Source: CAD feature listing. Evaluate the final solid. Frame: model axes, mm. Face numbers are marked on the shaded views. A direction names the side the tool comes from. Coordinates: 2 decimals unless noted, no trailing zeros. Order: outer loops, then holes, each group sorted by start corner. A loop starts at its lowest first (then second) coordinate and runs counter-clockwise, first axis right, second up. Notation, with made-up numbers: (-7, 44) - (-1, 44) arc R12 cw to (-1, 58) - close; hole circle Ø6 at (47.5, -25.5). An arc over 180 degrees is marked (long way). One line per question, with ' | ' between items.
Autodesk Inventor part; units mm, degrees
ref_plane "YZ Plane" through (0, 0, 0) normal (1, 0, 0) x (0, 1, 0)
ref_plane "XZ Plane" through (0, 0, 0) normal (0, 1, 0) x (-1, 0, 0)
ref_plane "XY Plane" through (0, 0, 0) normal (0, 0, 1) x (1, 0, 0)
sketch "Sketch1" plane through (0, 0, 0) normal (1, 0, 0) x (0, 1, 0)
  circle A0 centre (0, 0) radius 3.175
  circle A1 centre (0, 0) radius 6.35
  dimension "d0" = 6.35
  dimension "d1" = 12.7
extrude "Extrusion1" add sketch "Sketch1" along normal blind 25.4
sketch "Sketch2" plane through (25.4, 0, 0) normal (1, 0, 0) x (0, 0, -1)
  circle A0 centre (0, 0) radius 6.35
  circle A1 centre (0, 0) radius 1.5875
  circle A2 centre (0, 0) radius 6.35
  dimension "d4" = 3.175
extrude "Extrusion2" add sketch "Sketch2" along normal blind 12.7
sketch "Sketch3" plane through (38.1, 0, 0) normal (1, 0, 0) x (0, 0, -1)
  circle A0 centre (0, 0) radius 6.35
  line L0 (2, 16.0268) -> (2, 6.0268)
  line L1 (2, 16.0268) -> (6, 16.0268)
  line L2 (6, 16.0268) -> (6, 2.0791)
  line L3 (-2, 16.0268) -> (-2, 6.0268)
  line L4 (-2, 16.0268) -> (-6, 16.0268)
  line L5 (-6, 16.0268) -> (-6, 2.0791)
  dimension "d11" = 4
  dimension "d12" = 10
  dimension "d13" = 10
extrude "Extrusion3" add sketch "Sketch3" against normal blind 18 contours A0 L0 L1 L2 | L5 L4 L3 A0
chamfer "Chamfer1" distance 9 angle 45 2 edges at (20.1, 16.0268, 4) (20.1, 16.0268, -4)
chamfer "Chamfer2" distance 2 angle 45 2 edges at (38.1, 16.0268, 4) (38.1, 16.0268, -4)
sketch "Sketch5" plane through (20.1, 2.0791, 6) normal (0, 0, 1) x (1, 0, 0)
  line L0 (16, 13.9478) -> (9, 13.9478)
  line L1 (18, 11.9478) -> (18, 0)
  circle A0 centre (13, 8.9478) radius 0.75
  point P0 (-20.1, -2.0791)
  dimension "d30" = 1.5
  dimension "d31" = 5
  dimension "d32" = 5
extrude "Extrusion5" cut sketch "Sketch5" against normal blind 15
sketch "Sketch6" plane through (38.1, 0, 0) normal (1, 0, 0) x (0, 0, -1)
  arc A0 (2, 6.0268) -> (-2, 6.0268) centre (0, 0) ccw
  line L0 (-6, 14.0268) -> (-6, 2.0791)
  line L1 (2, 6.0268) -> (-2, 6.0268)
  point P0 (-6, 3.4641)
extrude "Extrusion6" cut sketch "Sketch6" against normal blind 6
pattern_circular "Circular Pattern3" count 3 over 360 about axis through (0, 0, 0) along (1, 0, 0) of "Extrusion3", "Chamfer2", "Extrusion5", "Extrusion6", "Chamfer1"
sketch "Sketch7" plane through (38.1, 0, 0) normal (1, 0, 0) x (0, 0, -1)
  circle A0 centre (0, 0) radius 1.5875
  circle A1 centre (0, 0) radius 1.524
  line L0 (-1.524, 1.524) -> (1.524, 1.524)
  line L1 (1.524, 1.524) -> (1.524, -1.524)
  line L2 (1.524, -1.524) -> (-1.524, -1.524)
  line L3 (-1.524, -1.524) -> (-1.524, 1.524)
  circle A2 centre (0, 0) radius 1.5875
  dimension "d43" = 3.048
extrude "Extrusion7" add sketch "Sketch7" against normal blind 3.175 contours A0 L1 | L1 A1 L0 A0 | A0 L2 A1 L1 | L0 A0 | A1 | A0 L2 | L0 A1 L3 A0 | L2 A0 L3 A1 | L3 A0
sketch "Sketch8" plane through (38.1, 0, 0) normal (1, 0, 0) x (0, 0, -1)
  line L0 (-1.651, 1.651) -> (1.651, 1.651)
  line L1 (1.651, 1.651) -> (1.651, -1.651)
  line L2 (1.651, -1.651) -> (-1.651, -1.651)
  line L3 (-1.651, -1.651) -> (-1.651, 1.651)
  point P0 (0, 0)
  dimension "d46" = 1.651
  dimension "d48" = 1.651
  dimension "d49" = 3.302
  dimension "d50" = 3.302
extrude "Extrusion8" cut sketch "Sketch8" against normal blind 12.7
properties part number "Coupler"
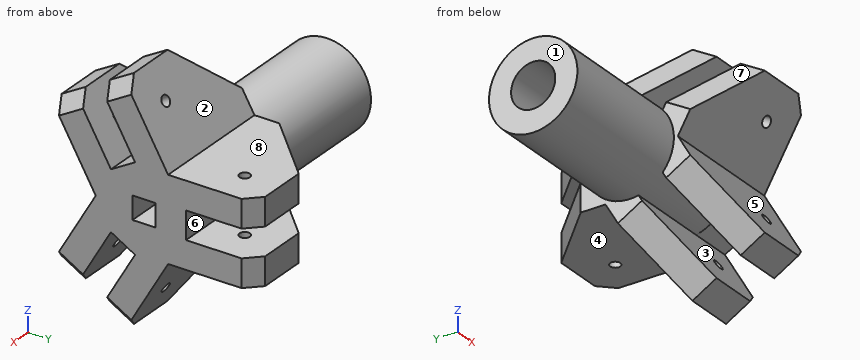
(1) Pull-direction query (Z, two-part tool) for the marked faces 1, 2 and 3; classes: pulls with the +Z half, pulls with the -Z half, needs draft (parallel to the pull), parting line crosses it, or undercut.
Taken from the geometry:
face 1: needs draft | face 2: pulls with the +Z half | face 3: undercut
(2) Pin query (flat end, axial travel): P1, Ø1, axis at x = 34.5, z = 0.5, coming from the +Y side; P2, Ø8, axis at x = 32, y = 9, coming from the +Z side; P3, Ø1.7, axis at x = 29, z = 0, coming from the -Y side. Return the tip coordinate at first contact, or that it passes through.
Taken from the geometry:
P1: stops at y = 6.03 | P2: stops at z = 6 | P3: stops at y = -7.42
(3) Cut plane B-B (z = -0.5). Return the cut outline in (x, y).
Taken from the geometry:
outline: (0, -6.33) - (20.1, -6.33) - (20.1, -7.22) - (38.1, -7.22) - (38.1, -1.65) - (25.4, -1.65) - (25.4, -3.14) - (0, -3.14) - close; (0, 3.14) - (25.4, 3.14) - (25.4, 1.65) - (38.1, 1.65) - (38.1, 6.03) - (32.1, 6.03) - (32.1, 6.33) - (0, 6.33) - close
(4) Cut plane D-D (z = 14). Return the cut outline in (x, y).
Taken from the geometry:
outline: (25.77, -1.15) - (28.08, -5.77) - (37.12, -5.77) - (38.1, -3.8) - (38.1, -1.15) - close
(5) Cut plane C-C (x = 26.5). Return the cut outline in (y, z), and give its area (3 significant figures).
Taken from the geometry:
outline: (-11.91, -8.63) - (-8.45, -10.63) - (-4.75, -4.22) arc R6.35 ccw to (-1.28, -6.22) - (-4.98, -12.63) - (-1.52, -14.63) - (3.46, -6) - (13.43, -6) - (13.43, -2) - (6.03, -2) arc R6.35 ccw to (6.03, 2) - (13.43, 2) - (13.43, 6) - (3.46, 6) - (-1.52, 14.63) - (-4.98, 12.63) - (-1.28, 6.22) arc R6.35 ccw to (-4.75, 4.22) - (-8.45, 10.63) - (-11.91, 8.63) - (-6.93, 0) - close; hole (-1.65, -1.65) - (1.65, -1.65) - (1.65, 1.65) - (-1.65, 1.65) - close | area: 324 mm²
(6) Set-up query: the marked faces 4, 5, 6, 7 and 8. Return all of +Z, -Z, +X, -X, +Y, -Y with unobstructed straight access to the full face (end or side cutting, diameter ignored); none if empty.
Taken from the geometry:
face 4: -Z, +X, -X, +Y | face 5: +X, -X, -Y | face 6: +X, +Y | face 7: +Z, -X, -Y | face 8: +Z, +X, -X, +Y
(7) Cut plane A-A (x = 31). Return the cut outline in (y, z).
Taken from the geometry:
outline: (-13.21, -10.88) - (-9.75, -12.88) - (-4.75, -4.22) arc R6.35 ccw to (-1.28, -6.22) - (-6.28, -14.88) - (-2.82, -16.88) - (3.46, -6) - (16.03, -6) - (16.03, -2) - (6.03, -2) arc R6.35 ccw to (6.03, 2) - (16.03, 2) - (16.03, 6) - (3.46, 6) - (-2.82, 16.88) - (-6.28, 14.88) - (-1.28, 6.22) arc R6.35 ccw to (-4.75, 4.22) - (-9.75, 12.88) - (-13.21, 10.88) - (-6.93, 0) - close; hole (-1.65, -1.65) - (1.65, -1.65) - (1.65, 1.65) - (-1.65, 1.65) - close
(8) Material intervals for L1, parallel to Z at x = 6.5, y = 0 (3 decimals); L2, parallel to Z at x = 29, y = 9.75; L3, parallel to X at y = -7.25, z = 8, sorted ascending. Write a range as from..to.
Taken from the geometry:
L1: z = -6.35..-3.175, 3.175..6.35 | L2: z = -6..-2, 2..6 | L3: x = 23.63..32.52, 33.68..38.1
